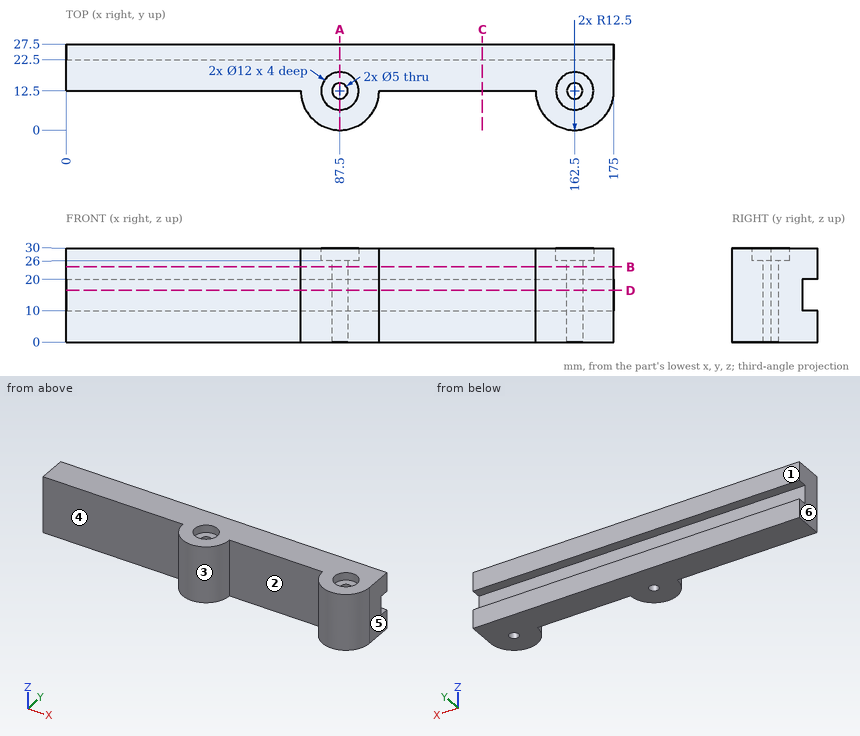
Print and shaded views of the part. All mm, measured from the part's lowest x, y and z. A direction names the side the tool comes from. Round coordinates to 2 decimals unless told otherwise and drop trailing zeros. Write each loop counter-clockwise with the first axis right and the second up, starting at its lowest first coordinate (ties: lowest second). Pieces come first, ordered by that corner, then holes. Notation, with made-up numbers: (69, 86.25) - (122, 86.25) arc R29 ccw to (122, 109.25) - close; hole circle Ø8 at (42, 42.5). An arc over 180 degrees is marked (long way). One line per item, written item: value.
(1) Drop flat-ended pins along their axis: P1, Ø8, axis at x = 65.5, z = 14, coming from the -Y side; P2, Ø6, axis at x = 164.5, y = 13, coming from the +Z side; P3, Ø6, axis at x = 138.5, z = 16.5, coming from the +Y side. Give the stop position or say it passes through.
Values follow:
P1: stops at y = 12.5
P2: stops at z = 26
P3: stops at y = 22.5
(2) Two-plate mould, pull along X, no slides. Class the marked faces 3, 4, 5 and 6: pulls with the +X half, pulls with the -X half, needs draft (parallel to the pull), parting line crosses it, or undercut.
Values follow:
face 3: undercut
face 4: needs draft
face 5: pulls with the +X half
face 6: pulls with the -X half
(3) Wall check: probe 1 along Y at (x, z) = (87.5, 7.75); probe 2 along Y at (x, z) = (162.5, 26.8); probe 3 along Z at (x, y) = (113.5, 23.25). Give the ranges that are in metal, low to high.
Values follow:
probe 1: y = 0 to 10, 15 to 27.5
probe 2: y = 0 to 6.5, 18.5 to 27.5
probe 3: z = 0 to 10, 20 to 30
(4) Cut at B-B, the plane z = 24. Give the cut face in (x, y), plus the area to 3 significant figures.
Values follow:
outline: (0, 12.5) - (75, 12.5) arc R12.5 ccw to (100, 12.5) - (150, 12.5) arc R12.5 ccw to (175, 12.5) - (175, 27.5) - (0, 27.5) - close; hole circle Ø5 at (87.5, 12.5); hole circle Ø5 at (162.5, 12.5)
area: 3,080 mm²
(5) Cut at C-C, the plane x = 133. Give the cut face in (y, z).
Values follow:
outline: (12.5, 0) - (27.5, 0) - (27.5, 10) - (22.5, 10) - (22.5, 20) - (27.5, 20) - (27.5, 30) - (12.5, 30) - close
(6) Cut at D-D, the plane z = 16.5. Give the cut face in (x, y), plus the area to 3 significant figures.
Values follow:
outline: (0, 12.5) - (75, 12.5) arc R12.5 ccw to (100, 12.5) - (150, 12.5) arc R12.5 ccw to (175, 12.5) - (175, 22.5) - (0, 22.5) - close; hole circle Ø5 at (87.5, 12.5); hole circle Ø5 at (162.5, 12.5)
area: 2,200 mm²
(7) Cut at A-A, the plane x = 87.5. Give the cut face in (y, z).
Values follow:
outline: (0, 0) - (10, 0) - (10, 26) - (6.5, 26) - (6.5, 30) - (0, 30) - close; (15, 0) - (27.5, 0) - (27.5, 10) - (22.5, 10) - (22.5, 20) - (27.5, 20) - (27.5, 30) - (18.5, 30) - (18.5, 26) - (15, 26) - close
(8) 3-axis set-ups, long thin cutter, end or side, ignore diameter. For the marked faces 1 and 2: which of +Z, -Z, +X, -X, +Y, -Y reach the whole face in a straight line?
Values follow:
face 1: +Z, -Z, +X, -X, +Y
face 2: +Z, -Z, -Y
